Verification items for the finished model (mm, model axes). A direction names the side the tool comes from. Round coordinates to 2 decimals unless told otherwise and drop trailing zeros. Order: outer loops, then holes, each group sorted by start corner. A loop starts at its lowest first (then second) coordinate and runs counter-clockwise, first axis right, second up.
```python
from build123d import *

# Parameters (mm, degrees)
F0_W           = 80
F0_H           = 80
F1_DEPTH       = 5
F0_R           = 32.25
F2_DEPTH       = 1.7
F4_D           = 3
F4_CSINK_D     = 5.75
F4_CSINK_ANGLE = 90
F6_D           = 2.4
F7_R           = 3.9


with BuildPart() as f1:
    # F0 (on Top) → F1 (new body)
    with BuildSketch(Plane.XY):
        Rectangle(F0_W, F0_H)
        Polygon((-38.86, 29.335), (-38.86, 38.86), (-29.335, 38.86), (29.335, 38.86), (38.86, 38.86), (38.86, 29.335), (38.86, -29.335), (38.86, -38.86), (29.335, -38.86), (-29.335, -38.86), (-38.86, -38.86), (-38.86, -29.335), align=None, mode=Mode.SUBTRACT)
        Polygon((-29.335, 38.86), (-38.86, 38.86), (-38.86, 29.335), align=None)
        Polygon((38.86, 38.86), (29.335, 38.86), (38.86, 29.335), align=None)
        Polygon((38.86, -38.86), (38.86, -29.335), (29.335, -38.86), align=None)
        Polygon((-29.335, -38.86), (-38.86, -29.335), (-38.86, -38.86), align=None)
    extrude(amount=F1_DEPTH)

    # F0 (on Top) → F2 (join)
    with BuildSketch(Plane.XY):
        Polygon((29.335, 38.86), (-29.335, 38.86), (-38.86, 29.335), (-38.86, -29.335), (-29.335, -38.86), (29.335, -38.86), (38.86, -29.335), (38.86, 29.335), align=None)
        Circle(F0_R, mode=Mode.SUBTRACT)
    extrude(amount=F2_DEPTH)

    # F4 (through all)
    with Locations(Plane.XY.offset(1.7)):
        with Locations((-25, 25), (25, 25), (25, -25), (-25, -25)):
            CounterSinkHole(F4_D / 2, F4_CSINK_D / 2, counter_sink_angle=F4_CSINK_ANGLE)

    # F6 (through all)
    with Locations(Plane.XY.offset(5)):
        with Locations((-35.685, 35.685), (35.685, 35.685), (35.685, -35.685), (-35.685, -35.685)):
            Hole(F6_D / 2)

    # F7
    f7_edges = [f1.edges().sort_by_distance(p)[0] for p in [
        (-40, -40, 2.5),
        (40, -40, 2.5),
        (40, 40, 2.5),
        (-40, 40, 2.5),
    ]]
    fillet(f7_edges, radius=F7_R)


solid = f1.part
```
1) Draft check along X on faces 3 (the cylindrical face through (26.11, 26.01, 0.16)), 4 (the cylindrical face through (-38.888, -38.827, 2.535)), 5 (the cylindrical face through (38.827, 38.888, 2.535)). Enter one of: released by +X, released by -X, zero draft, split by the parting line, or undercut.
2) Scan lines: probe 1 along Y at (x, z) = (-28.5, 3.7); probe 2 along Y at (x, z) = (25, 0.25). Record each from-to range of solid material in increasing order.
3) Go/stop test with flat-tipped pins: pin 1 Ø2 at (x, y) = (-35.685, -35.685) entering from -Z; pin 2 Ø5 at (x, y) = (-25, -25) entering from +Z (3 decimals); pin 3 Ø4 at (x, y) = (25, -25) entering from +Z (3 decimals). Record where each tip stops, or that it passes through.
4) Sectioned sample at C-C on y = -25. Record the cut outline in (x, z) (3 decimals).
5) Sectioned sample at A-A on x = 0. Record the cut outline in (y, z), then the cut area to 3 significant figures.
6) Tool access check on faces 1 (the cylindrical face through (-23.89, 26.01, 0.16)), 2 (the flat face through (-15, 29, 1.7)). Record the directions out of +Z, -Z, +X, -X, +Y, -Y that give a thin tool (end or side, any length) a straight path to the whole face; none if there is none.
Returned:
1. face 3: undercut
1. face 4: released by -X
1. face 5: released by +X
2. probe 1: y = -40 to -38.86, 38.86 to 40
2. probe 2: y = -40 to -26.5, -23.5 to -20.37, 20.37 to 23.5, 26.5 to 40
3. pin 1: passes through
3. pin 2: stops at z = 1.325
3. pin 3: stops at z = 0.825
4. outline: (-40, 0) - (-26.5, 0) - (-26.5, 0.325) - (-27.875, 1.7) - (-38.86, 1.7) - (-38.86, 5) - (-40, 5) - close; (-23.5, 0) - (-20.373, 0) - (-20.373, 1.7) - (-22.125, 1.7) - (-23.5, 0.325) - close; (20.373, 0) - (23.5, 0) - (23.5, 0.325) - (22.125, 1.7) - (20.373, 1.7) - close; (26.5, 0) - (40, 0) - (40, 5) - (38.86, 5) - (38.86, 1.7) - (27.875, 1.7) - (26.5, 0.325) - close
5. outline: (-40, 0) - (-32.25, 0) - (-32.25, 1.7) - (-38.86, 1.7) - (-38.86, 5) - (-40, 5) - close; (32.25, 0) - (40, 0) - (40, 5) - (38.86, 5) - (38.86, 1.7) - (32.25, 1.7) - close
5. area: 33.9 mm2
6. face 1: +Z, -Z
6. face 2: +Z
